from build123d import *

# Parameters (mm, degrees)
SKETCH_3_R          = 1.675
CUT_EXTRUDE_1_DEPTH = 10
SKETCH_4_R          = 1.75
CUT_EXTRUDE_2_DEPTH = 41.749233122
FILLET_1_R          = 1.5
SKETCH_5_R          = 25.75
SKETCH_5_R_2        = 23
EXTRUDE_1_DEPTH     = 21
EXTRUDE_START       = -4.1
SKETCH_7_R          = 25.75
SKETCH_7_R_2        = 18.5
EXTRUDE_2_DEPTH     = 4.1
EXTRUDE_START_2     = 1
SKETCH_8_R          = 25.75
SKETCH_8_R_2        = 17.5
EXTRUDE_3_DEPTH     = 1
FILLET_2_R          = 1
CHAMFER_1_SIZE      = 0.5


with BuildPart() as part:
    # 草图2 → 旋转1 (revolve)
    with BuildSketch(Plane(origin=(0, 0, 0), x_dir=(0, 0, -1), z_dir=(1, 0, 0)), mode=Mode.PRIVATE) as revolve_1_sk:
        Polygon((0, 0), (3, 0), (3, 16.036165005), (-13, 18.736165005), (-13, 26.5), (-16, 26.5), (-16, 16.2), (0, 13.5), align=None)
    revolve(revolve_1_sk.sketch.rotate(Axis((0, 0, 0), (0, 0, -1)), 90), axis=Axis((0, 0, 0), (0, 0, -1)))

    # 草图3 → 切除-拉伸1 (cut)
    with BuildSketch(Plane(origin=(0, 0, -3), x_dir=(-1, 0, 0), z_dir=(0, 0, -1))):
        with Locations((5.656854249, 5.656854249)):
            Circle(SKETCH_3_R)
        with Locations((5.656854249, -5.656854249)):
            Circle(SKETCH_3_R)
        with Locations((-5.656854249, 5.656854249)):
            Circle(SKETCH_3_R)
        with Locations((-5.656854249, -5.656854249)):
            Circle(SKETCH_3_R)
    extrude(amount=-CUT_EXTRUDE_1_DEPTH, mode=Mode.SUBTRACT)

    # 草图4 → 切除-拉伸2 (cut, through all)
    with BuildSketch(Plane(origin=(0, 0, 0), x_dir=(1, 0, 0), z_dir=(0, 1, 0))):
        with Locations(Location((0, -8, 0), (0, 0, 136.407373303))):
            Circle(SKETCH_4_R)
    extrude(amount=-CUT_EXTRUDE_2_DEPTH, mode=Mode.SUBTRACT)

    # 圆角1
    fillet_1_edges = [part.edges().sort_by_distance(p)[0] for p in [
        (-13.5, 0, 0),
        (-16.2, 0, 16),
        (-18.736165005, 0, 13),
        (-16.036165005, 0, -3),
    ]]
    fillet(fillet_1_edges, radius=FILLET_1_R)

    # 草图5 → 凸台-拉伸1 (add)
    with BuildSketch(Plane.XY.offset(16)):
        with Locations(Location((0, 0, 0), (0, 0, 180))):
            Circle(SKETCH_5_R)
        with Locations(Location((0, 0, 0), (0, 0, 180))):
            Circle(SKETCH_5_R_2, mode=Mode.SUBTRACT)
    extrude(amount=EXTRUDE_1_DEPTH)

    # 草图7 → 凸台-拉伸2 (add)
    with BuildSketch(Plane.XY.offset(37).offset(EXTRUDE_START)):
        with Locations(Location((0, 0, 0), (0, 0, 180))):
            Circle(SKETCH_7_R)
        Circle(SKETCH_7_R_2, mode=Mode.SUBTRACT)
    extrude(amount=EXTRUDE_2_DEPTH)

    # 草图8 → 凸台-拉伸3 (add)
    with BuildSketch(Plane(origin=(0, 0, 32.9), x_dir=(-1, 0, 0), z_dir=(0, 0, -1)).offset(EXTRUDE_START_2)):
        Circle(SKETCH_8_R)
        Circle(SKETCH_8_R_2, mode=Mode.SUBTRACT)
    extrude(amount=-EXTRUDE_3_DEPTH)

    # 圆角2
    fillet_2_edges = [part.edges().sort_by_distance(p)[0] for p in [
        (-26.5, 0, 13),
    ]]
    fillet(fillet_2_edges, radius=FILLET_2_R)

    # 倒角1
    chamfer_1_edges = [part.edges().sort_by_distance(p)[0] for p in [
        (-18.5, 0, 37),
    ]]
    chamfer(chamfer_1_edges, length=CHAMFER_1_SIZE)


solid = part.part
Verification items for the finished model (mm, model axes). A direction names the side the tool comes from. Give positions to 0.01 mm unless a question says otherwise; leave off trailing zeros. Loops run counter-clockwise (first coordinate to the right, second up) from the corner with the lowest first, then second, coordinate; pieces in that order, holes last. Notation, with made-up numbers: (59.25, 63.25) - (98.25, 63.25) arc R11 cw to (98.25, 77.25) - close; hole circle Ø3 at (31, 72.25). An arc over 180 degrees is marked (long way). Write each question's results on one line, items separated by ' | '.
1) Depth check by flat-ended pin: P1, Ø5.5, axis at x = -5.66, y = 5.66, coming from the -Z side; P2, Ø21, axis at x = 0, y = 0, coming from the +Z side; P3, Ø3, axis at y = 19, z = 12.5, coming from the -X side; P4, Ø8, axis at x = 20.5, z = 25.5, coming from the -Y side. Enter the tip coordinate at first touch or a pass-through.
Solution:
P1: z = -3 | P2: z = 0 | P3: x = -19.38 | P4: y = -19.77
2) Tool access check on faces 4 (the flat face through (5, -17, 16)), 5 (the flat face through (-11, 17, 13)), 6 (the flat face through (0, 0, 0)). Record the directions out of +Z, -Z, +X, -X, +Y, -Y that give a thin tool (end or side, any length) a straight path to the whole face; none if there is none.
Solution:
face 4: none | face 5: -Z | face 6: +Z
3) Sectioned sample at A-A on z = 19. Record the boundary of the cut face in (x, y), plus the area to 3 significant figures.
Solution:
outline: circle Ø51.5 at (0, 0); hole circle Ø46 at (0, 0) | area: 421 mm2
4) Sectioned sample at C-C on z = 5.5. Record the boundary of the cut face in (x, y).
Solution:
outline: circle Ø34.94 at (0, 0); hole circle Ø28.86 at (0, 0)
5) Sectioned sample at B-B on x = 6. Count the separate pieces of the cut face and the enclosed holes in it, plus the area to 3 significant figures.
Solution:
separate pieces: 3 | enclosed holes: 0 | area: 391 mm2
6) Mould release check, pull along Z, two halves, no side actions. Record for faces 1 (the flat face through (8.63, 15.44, 31.9)), 2 (the flat face through (11, -14, 32.9)), 3 (the cylindrical face through (-5.439, 7.318, -1.521)): pulls with the +Z half, pulls with the -Z half, needs draft (parallel to the pull), parting line crosses it, or undercut.
Solution:
face 1: undercut | face 2: pulls with the +Z half | face 3: needs draft
7) Material ranges on L1, parallel to Y at x = 0, z = 27.5; L2, parallel to Y at x = -7, z = 3.5; L3, parallel to X at y = -14, z = 29, recorded low to high. Write a range as from..to.
Solution:
L1: -25.75..-23, 23..25.75 | L2: -15.64..-12.23, 12.23..15.64 | L3: -21.61..-18.25, 18.25..21.61
